Geometry check sheet. Reference: the model listing, model coordinates, mm. A direction names the side the tool comes from. Coordinates: 2 decimals unless noted, no trailing zeros. Write each loop counter-clockwise with the first axis right and the second up, starting at its lowest first coordinate (ties: lowest second). Pieces come first, ordered by that corner, then holes. Notation, with made-up numbers: (17.25, -18) -> (74.25, -18) arc R23 ccw to (74.25, -6) -> close; hole circle Ø7 at (24.5, 44.5). An arc over 180 degrees is marked (long way). Use a Markdown table: item, result.
```python
from build123d import *

# Parameters (mm, degrees)
ESQUISSE2_W             = 150
ESQUISSE2_H             = 150
BOSS_EXTRU_1_DEPTH      = 5
ESQUISSE3_W             = 60
ESQUISSE3_H             = 12
ESQUISSE3_W_2           = 35
ENL_V_MAT_EXTRU_3_DEPTH = 107.183802908
ESQUISSE4_W             = 10
ESQUISSE4_H             = 10
ENL_V_MAT_EXTRU_4_DEPTH = 10


with BuildPart() as part:
    # Esquisse2 → Boss.-Extru.1 (new body)
    with BuildSketch(Plane.XY):
        Rectangle(ESQUISSE2_W, ESQUISSE2_H)
    extrude(amount=BOSS_EXTRU_1_DEPTH)

    # Esquisse3 → Enlèv. mat.-Extru.3 (cut, through all)
    with BuildSketch(Plane.XY.offset(5)):
        with Locations((5, 49)):
            Rectangle(ESQUISSE3_W, ESQUISSE3_H)
        with Locations((5, -49)):
            Rectangle(ESQUISSE3_W, ESQUISSE3_H)
        with Locations((-52.5, 0)):
            Rectangle(ESQUISSE3_W_2, ESQUISSE3_H)
    extrude(amount=-ENL_V_MAT_EXTRU_3_DEPTH, mode=Mode.SUBTRACT)

    # Esquisse4 → Enlèv. mat.-Extru.4 (cut)
    with BuildSketch(Plane.XY.offset(5)):
        with Locations((55, 0)):
            Rectangle(ESQUISSE4_W, ESQUISSE4_H)
    extrude(amount=-ENL_V_MAT_EXTRU_4_DEPTH, mode=Mode.SUBTRACT)


solid = part.part
```
Item 1: Section check A-A on x = 2.5. Record the boundary of the cut face in (y, z), then the cut area to 3 significant figures.
Answer block:
| item | result |
|---|---|
| outline | (-75, 0) -> (-55, 0) -> (-55, 5) -> (-75, 5) -> close; (-43, 0) -> (43, 0) -> (43, 5) -> (-43, 5) -> close; (55, 0) -> (75, 0) -> (75, 5) -> (55, 5) -> close |
| area | 630 mm^2 |
Item 2: Section check C-C on x = -46. Record the boundary of the cut face in (y, z), then the cut area to 3 significant figures.
Answer block:
| item | result |
|---|---|
| outline | (-75, 0) -> (-6, 0) -> (-6, 5) -> (-75, 5) -> close; (6, 0) -> (75, 0) -> (75, 5) -> (6, 5) -> close |
| area | 690 mm^2 |
Item 3: Thickness scan on L1, parallel to Y at x = 22.5, z = 0.25; L2, parallel to X at y = -4, z = 1.5; L3, parallel to Y at x = -51.5, z = 0.4. Record the ranges inside material, lowest first. Write a range as [from, to].
Answer block:
| item | result |
|---|---|
| L1 | y = [-75, -55], [-43, 43], [55, 75] |
| L2 | x = [-75, -70], [-35, 50], [60, 75] |
| L3 | y = [-75, -6], [6, 75] |
Item 4: Mould release check, pull along X, two halves, no side actions. Record for faces 1 (the flat face through (-75, -1, 2)), 2 (the flat face through (75, -1, 2)), 3 (the flat face through (-25, -49, 3)): +X half, -X half, draft (parallel to the pull), parting line (faces both ways), or undercut.
Answer block:
| item | result |
|---|---|
| face 1 | -X half |
| face 2 | +X half |
| face 3 | undercut |
Item 5: Tool access check on faces 4 (the flat face through (55, -5, 3)), 5 (the flat face through (-1, 1, 5)). Record the directions out of +Z, -Z, +X, -X, +Y, -Y that give a thin tool (end or side, any length) a straight path to the whole face; none if there is none.
Answer block:
| item | result |
|---|---|
| face 4 | +Z, -Z |
| face 5 | +Z, +X, -X, +Y, -Y |
Item 6: Section check D-D on z = 2. Record the boundary of the cut face in (x, y).
Answer block:
| item | result |
|---|---|
| outline | (-75, -75) -> (75, -75) -> (75, 75) -> (-75, 75) -> close; hole (-70, -6) -> (-35, -6) -> (-35, 6) -> (-70, 6) -> close; hole (-25, -55) -> (35, -55) -> (35, -43) -> (-25, -43) -> close; hole (-25, 43) -> (35, 43) -> (35, 55) -> (-25, 55) -> close; hole (50, -5) -> (60, -5) -> (60, 5) -> (50, 5) -> close |
Item 7: Depth check by flat-ended pin: P1, Ø4, axis at x = 26.5, y = -37.5, coming from the -Z side. Enter the tip coordinate at first touch or a pass-through.
Answer block:
| item | result |
|---|---|
| P1 | stops at z = 0 |
Item 8: Section check B-B on y = 45. Record the boundary of the cut face in (x, z), then the cut area to 3 significant figures.
Answer block:
| item | result |
|---|---|
| outline | (-75, 0) -> (-25, 0) -> (-25, 5) -> (-75, 5) -> close; (35, 0) -> (75, 0) -> (75, 5) -> (35, 5) -> close |
| area | 450 mm^2 |
